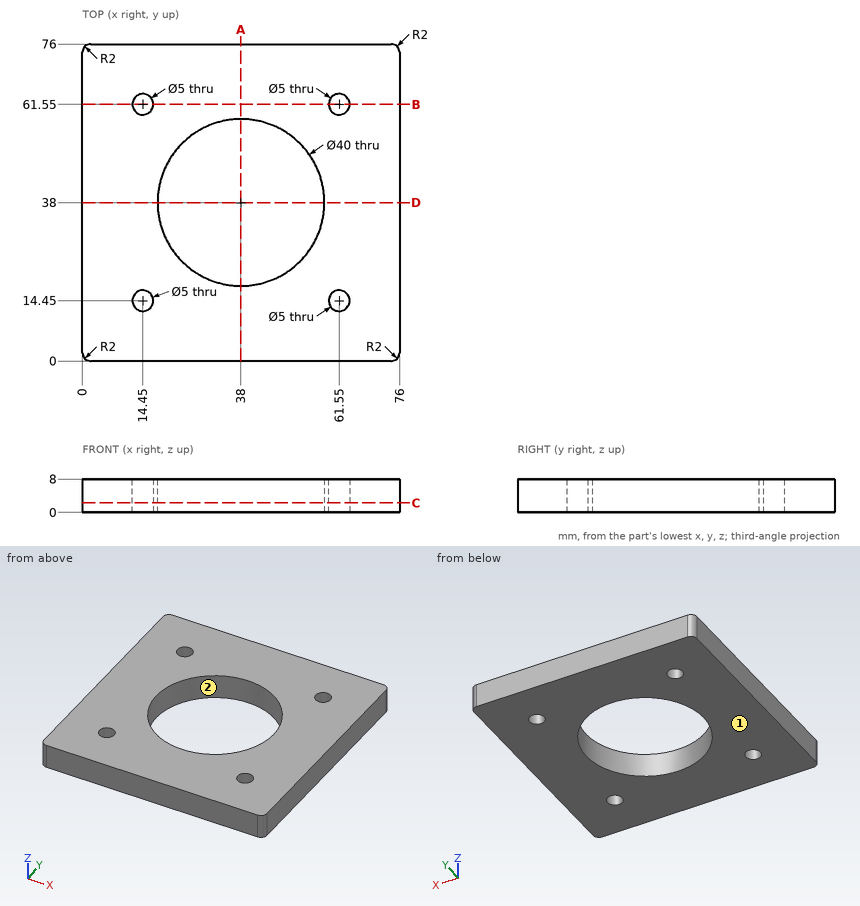
Design review of the part shown in the three views and the two pictorial views. Dimensions are in mm from the part's minimum x, y and z. Give positions to 0.01 mm unless a question says otherwise; leave off trailing zeros. Loops run counter-clockwise (first coordinate to the right, second up) from the corner with the lowest first, then second, coordinate; pieces in that order, holes last. Notation, with made-up numbers: (4.25, 49.25) -> (10.25, 49.25) arc R9 ccw to (10.25, 58.25) -> close; hole circle Ø4 at (74, 21.5). An arc over 180 degrees is marked (long way). Answer as a JSON object with one key per item and string values. Group by question number.
Q1. Take a section at B-B (y = 61.55). Write out the cut boundary in (x, z).
Q2. Take a section at C-C (z = 2.25). Write out the cut boundary in (x, y).
Q3. Take a section at A-A (x = 38). Write out the cut boundary in (y, z).
Q4. Wall thickness on line 1 along Y through (x, z) = (61.55, 5.75); line 2 along X through (y, z) = (61, 1.5); line 3 along X through (y, z) = (60, 4.75): over which ranges is each line inside the solid? List them lowest first.
Q5. Draft analysis for pull direction X (two halves, no side actions). For the marked faces 1 and 2, state which applies: pulls with the +X half, pulls with the -X half, needs draft (parallel to the pull), parting line crosses it, or undercut.
Q6. Insertion check: pin 1 (2 mm diameter, centred on y = 11, z = 4, fed in from -X). The pin has a flat end and moves straight along its axis. Give the tip position at first contact, or say it passes through.
Answer below:
{
 "1": {"outline": "(0, 0) -> (11.95, 0) -> (11.95, 8) -> (0, 8) -> close; (16.95, 0) -> (59.05, 0) -> (59.05, 8) -> (16.95, 8) -> close; (64.05, 0) -> (76, 0) -> (76, 8) -> (64.05, 8) -> close"},
 "2": {"outline": "(0, 2) arc R2 ccw to (2, 0) -> (74, 0) arc R2 ccw to (76, 2) -> (76, 74) arc R2 ccw to (74, 76) -> (2, 76) arc R2 ccw to (0, 74) -> close; hole circle Ø5 at (14.45, 14.45); hole circle Ø5 at (14.45, 61.55); hole circle Ø40 at (38, 38); hole circle Ø5 at (61.55, 14.45); hole circle Ø5 at (61.55, 61.55)"},
 "3": {"outline": "(0, 0) -> (18, 0) -> (18, 8) -> (0, 8) -> close; (58, 0) -> (76, 0) -> (76, 8) -> (58, 8) -> close"},
 "4": {"line 1": "y = 0 to 11.95, 16.95 to 59.05, 64.05 to 76", "line 2": "x = 0 to 12.01, 16.89 to 59.11, 63.99 to 76", "line 3": "x = 0 to 12.49, 16.41 to 59.59, 63.51 to 76"},
 "5": {"face 1": "needs draft", "face 2": "undercut"},
 "6": {"pin 1": "stops at x = 0"}
}
